Geometry check sheet. Reference: drawing and pictorial views, mm from the part's lowest x, y, z. A direction names the side the tool comes from. Give positions to 0.01 mm unless a question says otherwise; leave off trailing zeros. Order: outer loops, then holes, each group sorted by start corner. A loop starts at its lowest first (then second) coordinate and runs counter-clockwise, first axis right, second up. Notation, with made-up numbers: M 3.5,8 L 54.5,8 A17 ccw 54.5,37 Z; hole C 4,4 d7. An arc over 180 degrees is marked long. Answer as a JSON object with one key per item and string values. Group by question number.
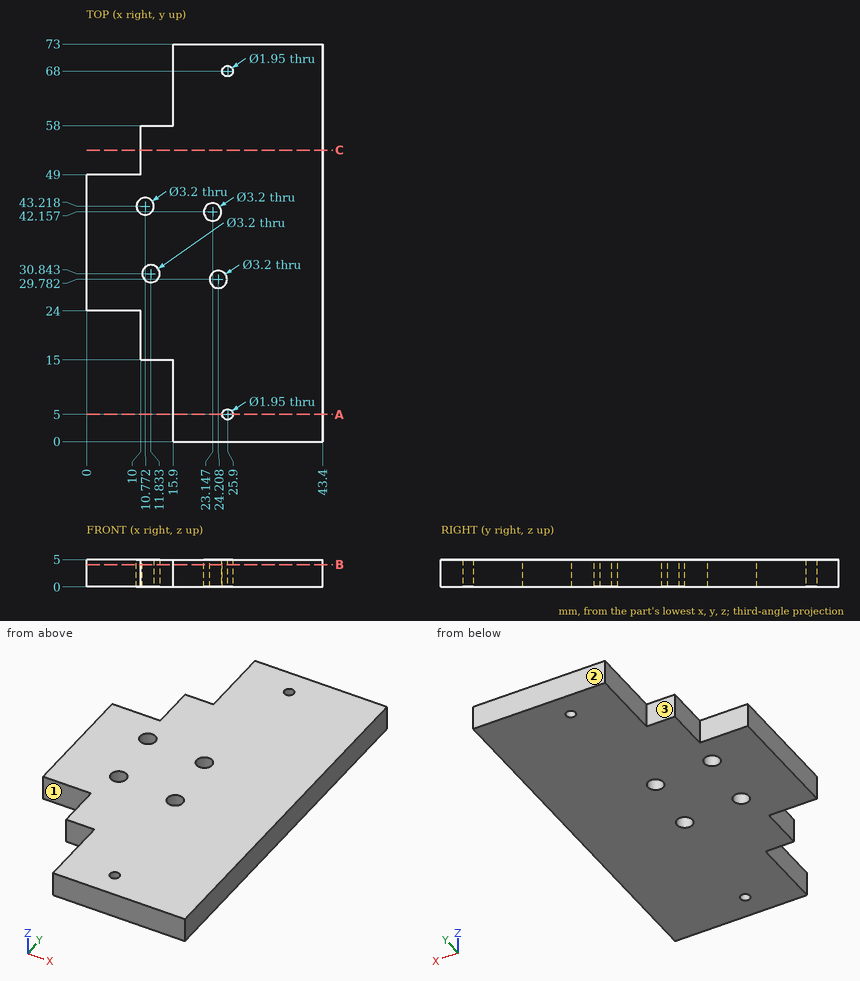
1. Access from +Z, -Z, +X, -X, +Y, -Y to the whole of each face (thin tool, end or side, straight path). Record for the marked faces 1, 2 and 3.
2. Cross-section at B-B (z = 4.1). State how many separate pieces and enclosed holes the cut face has, and give its area (3 significant figures).
3. Cross-section at C-C (y = 53.5). Record the cut outline in (x, z).
4. Thickness scan on line 1 along Y through (x, z) = (8, 1.65); line 2 along X through (y, z) = (10, 4); line 3 along X through (y, z) = (16.5, 1.8). Record the ranges inside material, lowest first. Write a range as [from, to].
5. Depth check by flat-ended pin: pin 1 (2.5 mm diameter, centred on y = 5.5, z = 2.5, fed in from -X); pin 2 (2.5 mm diameter, centred on x = 7, z = 2.5, fed in from -Y). Enter the tip coordinate at first touch or a pass-through.
6. Cross-section at A-A (y = 5). Record the cut outline in (x, z) (1 decimal), and give its area (3 significant figures).
Report:
{
 "1": {"face 1": "+Z, -Z, -X, -Y", "face 2": "+Z, -Z, +X, -X, +Y", "face 3": "+Z, -Z, -X, +Y"},
 "2": {"separate pieces": "1", "enclosed holes": "6", "area": "2,470 mm2"},
 "3": {"outline": "M 10,0 L 43.4,0 L 43.4,5 L 10,5 Z"},
 "4": {"line 1": "y = [24, 49]", "line 2": "x = [15.9, 43.4]", "line 3": "x = [10, 43.4]"},
 "5": {"pin 1": "stops at x = 15.9", "pin 2": "stops at y = 24"},
 "6": {"outline": "M 15.9,0 L 24.9,0 L 24.9,5 L 15.9,5 Z; M 26.9,0 L 43.4,0 L 43.4,5 L 26.9,5 Z", "area": "128 mm2"}
}
